Design review of the part built by this model. Coordinates are the model's own, in mm. Coordinates: 2 decimals unless noted, no trailing zeros. Write each loop counter-clockwise with the first axis right and the second up, starting at its lowest first coordinate (ties: lowest second). Pieces come first, ordered by that corner, then holes.
Q1. Take a section at B-B, the plane x = -371. Write out the cut boundary in (y, z) (3 decimals), plus the area to 3 significant figures.
Q2. For pin 1 Ø1 at (x, z) = (-433.5, 1) entering from -Y; pin 2 Ø1 at (x, z) = (22.5, 2) entering from +Y; pin 3 Ø1.6 at (x, z) = (17.5, 1.5) entering from +Y, all flat-tipped, find the tip position at first contact; note any pin that passes through.
Q3. Take a section at A-A, the plane x = -112.5. Write out the cut boundary in (y, z) (3 decimals).
Q4. For L1, parallel to Y at x = 109.5, z = 1.05; L2, parallel to Y at x = 7.5, z = 2.8, list the stretches that pass through material, from the lowest coordinate up.
from build123d import *

# Parameters (mm, degrees)
BOSS_EXTRUDE1_DEPTH = 3.175
CUT_EXTRUDE1_DEPTH  = 4.175
CUT_EXTRUDE2_DEPTH  = 7.62


with BuildPart() as part:
    # Sketch1 → Boss-Extrude1 (new body)
    with BuildSketch(Plane.XY):
        Polygon((-950.530495659, 69.619322302), (-951.061849964, 63.291592645), (-11.536706102, -24.902638492), (-8.372841274, -25.168315645), (0, -25.545856054), (152.4, -25.545856054), (152.4, -7.765856054), (139.7, -7.765856054), (139.7, -12.845856054), (136.525, -12.845856054), (136.525, -7.765856054), (95.25, -7.765856054), (95.25, -12.845856054), (92.075, -12.845856054), (92.075, -7.765856054), (79.375, -7.765856054), (79.375, -12.845856054), (76.2, -12.845856054), (76.2, -7.765856054), (69.85, -7.765856054), (25.4, -0.145856054), (19.05, -0.145856054), (19.05, -5.225856054), (15.875, -5.225856054), (15.875, -0.145856054), (3.175, -0.145856054), (3.175, -6.495856054), (0, -6.495856054), (0, -0.145856054), (-2.81225704, -0.145856054), (-6.247424053, 0.14260298), (-6.778778359, -6.185126677), (-9.942643187, -5.919449524), (-9.411288881, 0.408280132), (-946.54805097, 79.101852726), (-947.366630831, 69.353645149), align=None)
    extrude(amount=BOSS_EXTRUDE1_DEPTH)

    # Sketch2 → Cut-Extrude1 (cut, through all)
    with BuildSketch(Plane.XY.offset(3.175)):
        Polygon((-869.047169109, 67.116306724), (-868.590421605, 72.555567687), (-871.754286433, 72.821244839), (-872.210759203, 67.385255598), align=None)
        Polygon((-790.083960364, 60.403342827), (-789.620355495, 65.924265958), (-792.784220323, 66.189943111), (-793.247550458, 60.672291701), align=None)
        Polygon((-711.120751618, 53.69037893), (-710.650289385, 59.29296423), (-713.814154213, 59.558641383), (-714.284341712, 53.959327804), align=None)
        Polygon((-632.157542872, 46.977415032), (-631.680223276, 52.661662502), (-634.844088104, 52.927339654), (-635.321132966, 47.246363906), align=None)
        Polygon((-553.194334126, 40.264451135), (-552.710157166, 46.030360773), (-555.874021994, 46.296037926), (-556.35792422, 40.533400009), align=None)
        Polygon((-474.23112538, 33.551487238), (-473.740091056, 39.399059045), (-476.903955884, 39.664736197), (-477.394715474, 33.820436112), align=None)
        Polygon((-395.267916634, 26.83852334), (-394.770024946, 32.767757316), (-397.933889774, 33.033434469), (-398.431506728, 27.107472214), align=None)
        Polygon((-316.304707888, 20.125559443), (-315.799958836, 26.136455588), (-318.963823664, 26.402132741), (-319.468297982, 20.394508317), align=None)
        Polygon((-237.341499142, 13.412595546), (-236.829892727, 19.50515386), (-239.993757555, 19.770831012), (-240.505089236, 13.68154442), align=None)
        Polygon((-158.378290396, 6.699631648), (-157.859826617, 12.873852131), (-161.023691445, 13.139529284), (-161.54188049, 6.968580522), align=None)
        Polygon((-79.415081651, -0.013332249), (-78.889760507, 6.242550403), (-82.053625335, 6.508227555), (-82.578671745, 0.255616625), align=None)
    extrude(amount=-CUT_EXTRUDE1_DEPTH, mode=Mode.SUBTRACT)

    # Sketch3 → Cut-Extrude2 (cut)
    with BuildSketch(Plane.XY.offset(3.175)):
        Polygon((-435.836990415, 36.216246757), (-435.836990415, 26.451619727), (-427.115588921, 26.451619727), (-427.115588921, 14.108196169), (-989.316849096, 0), (-981.213716068, 132.265755076), align=None)
    extrude(amount=-CUT_EXTRUDE2_DEPTH, mode=Mode.SUBTRACT)


solid = part.part
Responses:
1. outline: (8.841, 0) - (30.772, 0) - (30.772, 3.175) - (8.841, 3.175) - close
1. area: 69.6 mm2
2. pin 1: stops at y = 26.45
2. pin 2: stops at y = -0.15
2. pin 3: stops at y = -5.23
3. outline: (-15.425, 0) - (9.065, 0) - (9.065, 3.175) - (-15.425, 3.175) - close
4. L1: y = -25.55 to -7.77
4. L2: y = -25.55 to -0.15
